Autodesk Inventor part; units mm, degrees
ref_plane "YZ Plane" through (0, 0, 0) normal (1, 0, 0) x (0, 1, 0)
ref_plane "XZ Plane" through (0, 0, 0) normal (0, 1, 0) x (-1, 0, 0)
ref_plane "XY Plane" through (0, 0, 0) normal (0, 0, 1) x (1, 0, 0)
sketch "Skizze1" plane through (0, 0, 0) normal (0, 0, 1) x (1, 0, 0)
  line L0 (0, 0) -> (0, 4)
  line L1 (0, 4) -> (9.5, 4)
  line L2 (9.5, 4) -> (9.5, 6)
  line L3 (9.5, 6) -> (61.5, 6)
  line L4 (61.5, 6) -> (61.5, 4)
  line L5 (61.5, 4) -> (71, 4)
  line L6 (71, 4) -> (71, 0)
  line L7 (71, 0) -> (0, 0)
  dimension "d1" = 9.5
  dimension "d2" = 9.5
  dimension "d3" = 8
  dimension "d4" = 12
  dimension "d29" = 52
revolve "Umdrehung1" add sketch "Skizze1" angle 360 about axis through (71, 0, 0) along (-1, 0, 0)
sketch "Skizze2" plane through (0, 0, 0) normal (-1, 0, 0) x (0, 0, 1)
  point P0 (0, 0)
  point P1 (0, 0)
sketch "Skizze3" plane through (71, 0, 0) normal (1, 0, 0) x (0, 0, -1)
  point P0 (0, 0)
  point P1 (0, 0)
hole "Bohrung1" at (71, 0, 0) direction (-1, 0, 0) diameter 4.134 depth 10 tip angle 118
hole "Bohrung2" at (0, 0, 0) direction (1, 0, 0) diameter 4.134 depth 10 tip angle 118
chamfer "Fase1" distance 0.5 angle 45 4 edges at (0, -4, 0) (71, -4, 0) (71, 0, 2.067) (0, 0, -2.067)
chamfer "Fase2" distance 0.1 angle 45 2 edges at (61.5, -6, 0) (9.5, -6, 0)
equation "\"d1\" = d2"
equation "\"d29\" = MainAxis_Schluesselweite + 2 * ParallelMech_Distance_Step2Flat"
equation "\"Flansch_ParralelMech_FlatPart_Width\" = 115"
properties part number "ParallelSystem_ProximalPart_Querstreben_v2" material "Edelstahl"
Source: CAD feature listing. Evaluate the final solid. Frame: model axes, mm. A direction names the side the tool comes from. Coordinates: 2 decimals unless noted, no trailing zeros. Loops run counter-clockwise (first coordinate to the right, second up) from the corner with the lowest first, then second, coordinate; pieces in that order, holes last. Notation, with made-up numbers: (-26, 46.5) - (27, 46.5) arc R18 ccw to (27, 71.5) - close; hole circle Ø5 at (-10, -8.75). An arc over 180 degrees is marked (long way). Return JSON: item names as keys, results as strings.
Q1. Mould query, pull axis Y, two halves, no side actions, for faces 4 (the flat face through (0, -2, -2)), 5 (the cylindrical face through (5.063, -0.867, -3.905)), 6 (the conical face through (59.974, -0.35, 0.078)). Classes: released by +Y, released by -Y, zero draft, split by the parting line, or undercut.
Results:
{"face 4": "zero draft", "face 5": "split by the parting line", "face 6": "undercut"}
Q2. Access query for faces 1 (the cylindrical face through (36, -6, 0)), 2 (the cylindrical face through (5.32, 1.26, -1.64)), 3 (the cylindrical face through (65.68, 1.26, 1.64)). Directions: +Z, -Z, +X, -X, +Y, -Y. A direction counts if a zero-diameter tool reaches every point of the face in a straight line with its end or side. Return the directions, or none.
Results:
{"face 1": "+X, -X", "face 2": "-X", "face 3": "+X"}
Q3. Section B-B, the plane x = 27. Return loops of the section in (y, z), plus the area to 3 significant figures.
Results:
{"outline": "circle Ø12 at (0, 0)", "area": "113 mm2"}
Q4. Section A-A, the plane x = 5.5. Return loops of the section in (y, z).
Results:
{"outline": "circle Ø8 at (0, 0); hole circle Ø4.13 at (0, 0)"}
Q5. Contact query for flat-ended pins moving along their axis: P1, Ø1, axis at x = 25.5, y = 4, coming from the +Z side; P2, Ø1.5, axis at x = 16, y = -1, coming from the -Z side; P3, Ø4, axis at x = 17, z = -3, coming from the +Y side. Output: stop coordinate, or through.
Results:
{"P1": "z = 4.87", "P2": "z = -5.99", "P3": "y = 5.92"}
Q6. Material intervals for line 1 along Y through (x, z) = (66.75, 0); line 2 along Z through (x, y) = (39.5, -0.25), sorted ascending.
Results:
{"line 1": "-4 to -2.07, 2.07 to 4", "line 2": "-5.99 to 5.99"}
